Can you work these out from the model? Positions are in its coordinate system, mm. Give positions to 0.01 mm unless a question says otherwise; leave off trailing zeros. Order: outer loops, then holes, each group sorted by start corner. A loop starts at its lowest first (then second) coordinate and runs counter-clockwise, first axis right, second up. Notation, with made-up numbers: (10.5, 27.25) - (58.5, 27.25) arc R21 cw to (58.5, 41.25) - close; hole circle Ø5 at (23.5, -7.5). An arc over 180 degrees is marked (long way). Answer as a JSON object with one key per item and string values.
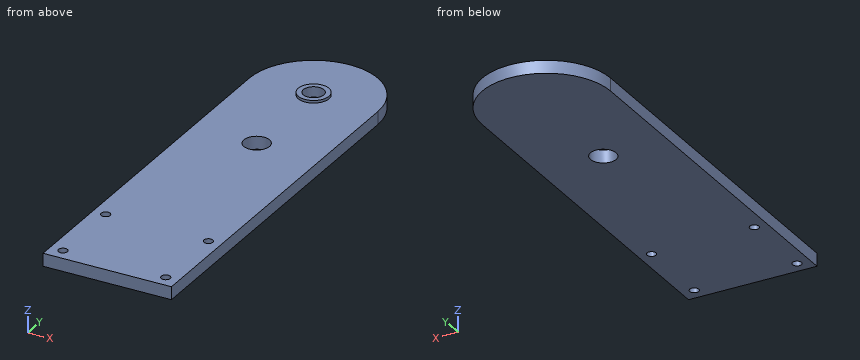
```python
from build123d import *

# Parameters (mm, degrees)
BOSS_EXTRUDE1_DEPTH = 5
SKETCH2_R           = 4
CUT_EXTRUDE1_DEPTH  = 3
BOSS_EXTRUDE2_START = 1
SKETCH3_R           = 6
SKETCH3_R_2         = 4
BOSS_EXTRUDE2_DEPTH = 1
SKETCH4_R           = 1.75
CUT_EXTRUDE2_DEPTH  = 148.224318643
SKETCH5_R           = 5
CUT_EXTRUDE3_DEPTH  = 148.224318643


with BuildPart() as part:
    # Sketch1 → Boss-Extrude1 (new body)
    with BuildSketch(Plane.XY):
        with BuildLine():
            Line((-25, -145), (25, -145))
            Line((25, -145), (25, 0))
            ThreePointArc((25, 0), (0, 25), (-25, 0))
            Line((-25, 0), (-25, -145))
        make_face()
    extrude(amount=BOSS_EXTRUDE1_DEPTH)

    # Sketch2 → Cut-Extrude1 (cut)
    with BuildSketch(Plane.XY.offset(5)):
        Circle(SKETCH2_R)
    extrude(amount=-CUT_EXTRUDE1_DEPTH, mode=Mode.SUBTRACT)

    # Sketch3 → Boss-Extrude2 (add)
    with BuildSketch(Plane.XY.offset(5).offset(BOSS_EXTRUDE2_START)):
        Circle(SKETCH3_R)
        Circle(SKETCH3_R_2, mode=Mode.SUBTRACT)
    extrude(amount=-BOSS_EXTRUDE2_DEPTH)

    # Sketch4 → Cut-Extrude2 (cut, through all)
    with BuildSketch(Plane.XY.offset(5)):
        with Locations((-20, -140)):
            Circle(SKETCH4_R)
        with Locations((-20, -110)):
            Circle(SKETCH4_R)
        with Locations(Location((20, -110, 0), (0, 0, 180))):
            Circle(SKETCH4_R)
        with Locations(Location((20, -140, 0), (0, 0, 180))):
            Circle(SKETCH4_R)
    extrude(amount=-CUT_EXTRUDE2_DEPTH, mode=Mode.SUBTRACT)

    # Sketch5 → Cut-Extrude3 (cut, through all)
    with BuildSketch(Plane.XY.offset(5)):
        with Locations((0, -40)):
            Circle(SKETCH5_R)
    extrude(amount=-CUT_EXTRUDE3_DEPTH, mode=Mode.SUBTRACT)


solid = part.part
```
Q1. I need wall thicknesses on L1, parallel to X at y = -140, z = 1.85; L2, parallel to Y at x = 0, z = 3.2; L3, parallel to Y at x = -20, z = 1.95. Which ranges of each line are inside material? Lowest first, please.
Recorded:
{"L1": "x = -25 to -21.75, -18.25 to 18.25, 21.75 to 25", "L2": "y = -145 to -45, -35 to -4, 4 to 25", "L3": "y = -145 to -141.75, -138.25 to -111.75, -108.25 to 15"}
Q2. I'm going to push flat-ended pins straight in: pin 1 Ø2.5 at (x, y) = (1.5, 0) entering from +Z; pin 2 Ø4 at (x, y) = (-12, -40) entering from +Z; pin 3 Ø6 at (x, y) = (0, -40) entering from -Z. Where does each tip first touch, or does it pass through?
Recorded:
{"pin 1": "stops at z = 2", "pin 2": "stops at z = 5", "pin 3": "passes through"}
Q3. If we section it at B-B, the plane z = 1: Please give me the cut outline in (x, y).
Recorded:
{"outline": "(-25, -145) - (25, -145) - (25, 0) arc R25 ccw to (-25, 0) - close; hole circle Ø3.5 at (-20, -140); hole circle Ø3.5 at (-20, -110); hole circle Ø10 at (0, -40); hole circle Ø3.5 at (20, -140); hole circle Ø3.5 at (20, -110)"}
Q4. If we section it at D-D, the plane y = -140: Please give me the cut outline in (x, z), then the cut area to 3 significant figures.
Recorded:
{"outline": "(-25, 0) - (-21.75, 0) - (-21.75, 5) - (-25, 5) - close; (-18.25, 0) - (18.25, 0) - (18.25, 5) - (-18.25, 5) - close; (21.75, 0) - (25, 0) - (25, 5) - (21.75, 5) - close", "area": "215 mm^2"}
Q5. If we section it at A-A, the plane y = -40: Please give me the cut outline in (x, z).
Recorded:
{"outline": "(-25, 0) - (-5, 0) - (-5, 5) - (-25, 5) - close; (5, 0) - (25, 0) - (25, 5) - (5, 5) - close"}
Q6. If we section it at C-C, the plane x = -20: Please give me the cut outline in (y, z).
Recorded:
{"outline": "(-145, 0) - (-141.75, 0) - (-141.75, 5) - (-145, 5) - close; (-138.25, 0) - (-111.75, 0) - (-111.75, 5) - (-138.25, 5) - close; (-108.25, 0) - (15, 0) - (15, 5) - (-108.25, 5) - close"}
